Verification items for the finished model (mm, model axes). A direction names the side the tool comes from. Coordinates: 2 decimals unless noted, no trailing zeros. Order: outer loops, then holes, each group sorted by start corner. A loop starts at its lowest first (then second) coordinate and runs counter-clockwise, first axis right, second up. Notation, with made-up numbers: M 57.25,75.25 L 89.25,75.25 A17 cw 89.25,106.25 Z; hole C 6,68 d9. An arc over 180 degrees is marked long. Answer as a JSON object with one key per item and string values. Group by question number.
(1) Cross-section at B-B (z = 50). Enter the section's corners in (x, y), plus the area to 3 significant figures.
(2) Material ranges on line 1 (Z direction, x = 9.25, y = 83); line 2 (Z direction, x = 9, y = 31); line 3 (Y direction, x = 3, z = 71.5), recorded low to high.
(3) Cross-section at A-A (y = 26.5). Enter the section's corners in (x, z), plus the area to 3 significant figures.
(4) Cross-section at D-D (y = 36). Enter the section's corners in (x, z), plus the area to 3 significant figures.
(5) Gauge pin test, flat ends, axial feed: pin 1 Ø1.5 at (x, y) = (4, 24) entering from -Z; pin 2 Ø1 at (x, y) = (8, 20) entering from -Z; pin 3 Ø3 at (x, z) = (2.5, 144) entering from +Y. Record the tip position at first contact, or that the pin passes through.
(6) Access from +Z, -Z, +X, -X, +Y, -Y to the whole of each face (thin tool, end or side, straight path). Record for faces 5 (the face through (5.916, 35.598, 200.063)), 6 (the face through (6.08, 75.69, 234.63)), 7 (the face through (5.916, 27.749, -1.443)).
(7) Cross-section at C-C (y = 17). Enter the section's corners in (x, z).
(8) Mould release check, pull along Z, two halves, no side actions. Record for faces 1 (the face through (6.084, 51.744, 214.669)), 2 (the face through (5.916, 82.586, 214.44)), 3 (the face through (5.916, 63.416, 225.491)), 4 (the face through (6.08, 83.27, 225.59)): released by +Z, released by -Z, zero draft, split by the parting line, or undercut.
from build123d import *

# Parameters (mm, degrees)
AUFSATZ_LINEAR_AUSTRAGEN1_DEPTH = 12
AUFSATZ_LINEAR_AUSTRAGEN3_DEPTH = 12
AUFSATZ_LINEAR_AUSTRAGEN4_DEPTH = 12
SCHNITT_LINEAR_AUSTRAGEN1_DEPTH = 254.175024926
VERRUNDUNG1_R                   = 50
SKIZZE9_W                       = 12
SKIZZE9_H                       = 12
AUFSATZ_LINEAR_AUSTRAGEN6_DEPTH = 11
AUFSATZ_LINEAR_AUSTRAGEN7_DEPTH = 12
SKIZZE11_R                      = 1.75
SCHNITT_LINEAR_AUSTRAGEN3_DEPTH = 10
SKIZZE12_R                      = 2.75
SCHNITT_LINEAR_AUSTRAGEN4_DEPTH = 3.6
FASE1_SIZE                      = 1.5
SCHNITT_LINEAR_AUSTRAGEN8_DEPTH = 254.549622303


with BuildPart() as part:
    # Skizze1 → Aufsatz-Linear austragen1 (new body)
    with BuildSketch(Plane(origin=(0, 0, 0), x_dir=(0, 0, -1), z_dir=(1, 0, 0))):
        with BuildLine():
            Line((-240, 65), (-230.735708163, 72.773663864))
            ThreePointArc((-230.735708163, 72.773663864), (-123.944567763, 17.242039243), (-3.735818811, 23.403668612))
            Line((-3.735818811, 23.403668612), (0, 12))
            ThreePointArc((0, 12), (-127.247502729, 5.681119716), (-240, 65))
        make_face()
    extrude(amount=AUFSATZ_LINEAR_AUSTRAGEN1_DEPTH)

    # Skizze4 → Aufsatz-Linear austragen3 (add)
    with BuildSketch(Plane(origin=(0, 0, 0), x_dir=(0, 0, -1), z_dir=(1, 0, 0))):
        with BuildLine():
            Line((-3.735818811, 23.403668612), (6.769031275, 32.218284445))
            Line((6.769031275, 32.218284445), (14.482482591, 23.025751128))
            Line((14.482482591, 23.025751128), (2.225771501, 12.741149373))
            ThreePointArc((2.225771501, 12.741149373), (1.113785782, 12.367871772), (0, 12))
            Line((0, 12), (-3.735818811, 23.403668612))
        make_face()
    extrude(amount=AUFSATZ_LINEAR_AUSTRAGEN3_DEPTH)

    # Skizze5 → Aufsatz-Linear austragen4 (add)
    with BuildSketch(Plane(origin=(12, 0, 0), x_dir=(0, 0, -1), z_dir=(1, 0, 0))):
        Polygon((-231.662517154, 71.995978781), (-222.469983836, 79.709430098), (-210.899806862, 65.920630121), (-192.948331238, 44.526894555), (-220.092340179, 58.207178805), align=None)
    extrude(amount=-AUFSATZ_LINEAR_AUSTRAGEN4_DEPTH)

    # Skizze6 → Schnitt-Linear austragen1 (cut, through all)
    with BuildSketch(Plane(origin=(12, 0, 0), x_dir=(0, 0, -1), z_dir=(1, 0, 0))):
        Polygon((-231.662517154, 71.995978781), (-199.510648028, 33.678873242), (-204.367668784, 29.603348917), (-240, 65), align=None)
    extrude(amount=-SCHNITT_LINEAR_AUSTRAGEN1_DEPTH, mode=Mode.SUBTRACT)

    # Verrundung1
    verrundung1_edges = [part.edges().sort_by_distance(p)[0] for p in [
        (6, 44.526894555, 192.948331238),
        (6, 35.285406895, 200.858689823),
    ]]
    fillet(verrundung1_edges, radius=VERRUNDUNG1_R)

    # Skizze9 → Aufsatz-Linear austragen6 (add)
    with BuildSketch(Plane(origin=(0, 156.320496136, 131.168470653), x_dir=(1, 0, 0), z_dir=(0, 0.7660444431189836, 0.6427876096865328))):
        with Locations((6, -125.185660837)):
            Rectangle(SKIZZE9_W, SKIZZE9_H)
    extrude(amount=AUFSATZ_LINEAR_AUSTRAGEN6_DEPTH)

    # Skizze10 → Aufsatz-Linear austragen7 (add)
    with BuildSketch(Plane.ZY):
        with BuildLine():
            Line((231.662517154, 71.995978781), (237.790872699, 66.853677904))
            Line((237.790872699, 66.853677904), (233.93414704, 62.257411245))
            ThreePointArc((233.93414704, 62.257411245), (228.094600221, 64.098613285), (222.663490618, 61.271356578))
            Line((222.663490618, 61.271356578), (231.662517154, 71.995978781))
        make_face()
        with BuildLine():
            Line((213.470957301, 68.984807894), (222.469983836, 79.709430098))
            Line((222.469983836, 79.709430098), (216.341628291, 84.851730975))
            Line((216.341628291, 84.851730975), (212.484902633, 80.255464316))
            ThreePointArc((212.484902633, 80.255464316), (215.31215934, 74.824354713), (213.470957301, 68.984807894))
        make_face()
    extrude(amount=-AUFSATZ_LINEAR_AUSTRAGEN7_DEPTH)

    # Skizze11 → Schnitt-Linear austragen3 (cut)
    with BuildSketch(Plane(origin=(0, 156.320496136, 131.168470653), x_dir=(1, 0, 0), z_dir=(0, 0.7660444431189826, 0.642787609686534))):
        with Locations(Location((6, -115.785660837, 0), (0, 0, 270))):
            Circle(SKIZZE11_R)
        with Locations(Location((6, -134.585660837, 0), (0, 0, 270))):
            Circle(SKIZZE11_R)
    extrude(amount=-SCHNITT_LINEAR_AUSTRAGEN3_DEPTH, mode=Mode.SUBTRACT)

    # Skizze12 → Schnitt-Linear austragen4 (cut)
    with BuildSketch(Plane(origin=(0, 148.660051704, 124.740594556), x_dir=(1, 0, 0), z_dir=(0, 0.7660444431189826, 0.642787609686534))):
        with Locations((6, -134.585660837)):
            Circle(SKIZZE12_R)
        with Locations((6, -115.785660837)):
            Circle(SKIZZE12_R)
    extrude(amount=SCHNITT_LINEAR_AUSTRAGEN4_DEPTH, mode=Mode.SUBTRACT)

    # Fase1
    fase1_edges = [part.edges().sort_by_distance(p)[0] for p in [
        (6, 88.135918972, 229.540647543),
        (6, 80.422467656, 238.73318086),
    ]]
    chamfer(fase1_edges, length=FASE1_SIZE)

    # Skizze16 → Schnitt-Linear austragen8 (cut, through all)
    with BuildSketch(Plane(origin=(12, 0, 0), x_dir=(0, 0, -1), z_dir=(1, 0, 0))):
        Polygon((-222.469983836, 79.709430098), (-222.546588281, 79.645151337), (-228.717349334, 86.999177991), (-228.640744889, 87.063456752), align=None)
        Polygon((-237.833278207, 79.350005435), (-231.662517154, 71.995978781), (-231.585912709, 72.060257542), (-237.756673762, 79.414284196), align=None)
    extrude(amount=-SCHNITT_LINEAR_AUSTRAGEN8_DEPTH, mode=Mode.SUBTRACT)


solid = part.part
Taken from the geometry:
{
 "1": {"outline": "M 0,1.32 L 12,1.32 L 12,13.39 L 0,13.39 Z", "area": "145 mm²"},
 "2": {"line 1": "z = 214.79 to 218.55, 225.36 to 235.66", "line 2": "z = -7.79 to -5.32, 166.6 to 193.52", "line 3": "y = 0.03 to 12.03"},
 "3": {"outline": "M 0,-11.57 L 12,-11.57 L 12,0.05 L 0,0.05 Z; M 0,155.45 L 12,155.45 L 12,185.16 L 0,185.16 Z", "area": "496 mm²"},
 "4": {"outline": "M 0,177.35 L 12,177.35 L 12,200.54 L 0,200.54 Z", "area": "278 mm²"},
 "5": {"pin 1": "stops at z = -14.29", "pin 2": "stops at z = -11.47", "pin 3": "stops at y = 23.04"},
 "6": {"face 5": "+Z, +X, -X, -Y", "face 6": "+Z, +X, -X", "face 7": "+X, -X, +Y"},
 "7": {"outline": "M 0,-7.3 L 12,-7.3 L 12,27.53 L 0,27.53 Z; M 0,122.82 L 12,122.82 L 12,164.18 L 0,164.18 Z"},
 "8": {"face 1": "released by +Z", "face 2": "released by -Z", "face 3": "undercut", "face 4": "undercut"}
}
